Check sheet for the modelled part. Datum: model origin and axes. Units: mm. A direction names the side the tool comes from. Coordinates: 2 decimals unless noted, no trailing zeros. Loops run counter-clockwise (first coordinate to the right, second up) from the corner with the lowest first, then second, coordinate; pieces in that order, holes last.
```python
from build123d import *

# Parameters (mm, degrees)
BOX_W          = 1
BOX_H          = 10
BOX_DEPTH      = 2
CYLINDER_R     = 2
CYLINDER_DEPTH = 10


with BuildPart() as cub:
    # Box → Box (new body)
    with BuildSketch(Plane(origin=(-0.5, -5, 1), x_dir=(1, 0, 0), z_dir=(0, 0, 1))):
        with Locations((0.5, 5)):
            Rectangle(BOX_W, BOX_H)
    extrude(amount=BOX_DEPTH)


with BuildPart() as cilindre:
    # Cylinder → Cylinder (new body)
    with BuildSketch(Plane.XY.offset(-10)):
        Circle(CYLINDER_R)
    extrude(amount=CYLINDER_DEPTH)


with BuildPart() as cut:
    # Cone → Cone (revolve)
    with BuildSketch(Plane.XZ):
        Polygon((0, 0), (2, 0), (2.8, 2.2), (0, 2.2), align=None)
    revolve(axis=Axis((0, 0, 0), (0, 0, 1)))

    # Fusion: union Cilindre
    add(cilindre.part)

    # Cut: cut Cub
    add(cub.part, mode=Mode.SUBTRACT)


solid = cut.part
```
1) Mould release check, pull along X, two halves, no side actions. Record for faces 4 (the flat face through (0, 0, -10)), 5 (the flat face through (0, 0, 1)), 6 (the conical face through (-0.46, -2.09, 0.38)): +X half, -X half, draft (parallel to the pull), parting line (faces both ways), or undercut.
Answer sheet:
face 4: draft
face 5: undercut
face 6: parting line
2) Scan lines: line 1 (X direction, y = 2.15, z = 1.25); line 2 (Y direction, x = 0.05, z = -3.5); line 3 (Y direction, x = 0.45, z = -7). Record each from-to range of solid material in increasing order.
Answer sheet:
line 1: x = -1.18 to -0.5, 0.5 to 1.18
line 2: y = -2 to 2
line 3: y = -1.95 to 1.95
3) Section check A-A on y = 0. Enter the section's corners in (x, z), plus the area to 3 significant figures.
Answer sheet:
outline: (-2.8, 2.2) - (-2, 0) - (-2, -10) - (2, -10) - (2, 0) - (2.8, 2.2) - (0.5, 2.2) - (0.5, 1) - (-0.5, 1) - (-0.5, 2.2) - close
area: 49.4 mm2
4) Set-up check for faces 1 (the flat face through (-0.5, 0, 2)), 2 (the cylindrical face through (0, -2, -5)), 3 (the flat face through (1, 0, 2.2)): record each of +Z, -Z, +X, -X, +Y, -Y from which the full face is reachable in a straight line by a thin tool's end or side.
Answer sheet:
face 1: +Z, +Y, -Y
face 2: -Z
face 3: +Z, +X, -X, +Y, -Y
5) Section check C-C on z = -8.5. Enter the section's corners in (x, y).
Answer sheet:
outline: circle Ø4 at (0, 0)
6) Depth check by flat-ended pin: pin 1 (1.5 mm diameter, centred on y = -2, z = -4.5, fed in from -X); pin 2 (1 mm diameter, centred on y = -1.5, z = -8, fed in from +X). Enter the tip coordinate at first touch or a pass-through.
Answer sheet:
pin 1: stops at x = -1.56
pin 2: stops at x = 1.73
7) Section check B-B on x = 0. Enter the section's corners in (y, z).
Answer sheet:
outline: (-2.36, 1) - (-2, 0) - (-2, -10) - (2, -10) - (2, 0) - (2.36, 1) - close
